Part model, mm, in its own coordinate system. A direction names the side the tool comes from. Coordinates: 2 decimals unless noted, no trailing zeros. Write each loop counter-clockwise with the first axis right and the second up, starting at its lowest first coordinate (ties: lowest second). Pieces come first, ordered by that corner, then holes. Notation, with made-up numbers: M 1,-4.5 L 15,-4.5 A25 ccw 15,31.5 Z; hole C 31.25,-5 d3. An arc over 180 degrees is marked long. Use a Markdown table: item, result. Add a question column.
Q1. Slice it at A-A on y = 0. Write the cut outline in (x, z), then the cut area to 3 significant figures.
Q2. Tool access for faces 1 (the flat face through (-29, -23.812, 5)), 2 (the flat face through (5, 38.1, 23)), 3 (the flat face through (18.149, 11.414, 5.478)), 4 (the flat face through (29, -23.812, 5)): list every direction of +Z, -Z, +X, -X, +Y, -Y with a clear straight run to the whole face (end or side of a thin tool).
Q3. Slice it at C-C on x = 8. Write the cut outline in (y, z), then the cut area to 3 significant figures.
Q4. Mould opens along X. For faces 5 (the cylindrical face through (-0.419, 44.361, 52.383)), 6 (the flat face through (34.925, -29, 5)), 7 (the flat face through (-2.63, 44.45, 38.43)) say: released by +X, released by -X, zero draft, split by the parting line, or undercut.
Q5. Pin check, flat tips, straight feed: pin 1 Ø12.5 at (y, z) = (38, 24.5) entering from +X; pin 2 Ø1 at (x, y) = (22, -2) entering from -Z; pin 3 Ø6 at (x, y) = (-13.5, 29) entering from +Z; pin 4 Ø24.5 at (x, z) = (5.5, 35.5) entering from -Y. Stop position of each tip, or through.
Q6. Wall check: L1, parallel to Z at x = 0, y = 48; L2, parallel to Z at x = 0, y = 40 (3 decimals); L3, parallel to Y at x = 0, z = 4. Give the ranges that are in metal, low to high. Write a range as from..to.
Q7. Slice it at B-B on x = 0. Count the separate pieces of the cut face and the enclosed holes in it, then the cut area to 3 significant figures.
from build123d import *

# Parameters (mm, degrees)
PAD_DEPTH       = 11.1125
PAD001_DEPTH    = 12.7
SKETCH002_R     = 11.1125
POCKET_DEPTH    = 6.35
SKETCH003_R     = 5.55625
POCKET001_DEPTH = 6.351


with BuildPart() as part:
    # Sketch → Pad (new body)
    with BuildSketch(Plane.XY):
        with BuildLine():
            ThreePointArc((4.957324, 11.692516), (-8.980256, -8.980256), (11.692516, 4.957324))
            Line((24.428163, 17.692971), (11.692516, 4.957324))
            ThreePointArc((23.688223, -18.672024), (30.156258, -0.613607), (24.428163, 17.692971))
            ThreePointArc((23.688223, -18.672024), (23.325058, -22.023177), (26.181706, -23.8125))
            Line((31.75, -23.8125), (26.181706, -23.8125))
            ThreePointArc((34.925, -26.9875), (33.995064, -24.742436), (31.75, -23.8125))
            Line((34.925, -31.75), (34.925, -26.9875))
            Line((-34.925, -31.75), (34.925, -31.75))
            Line((-34.925, -31.75), (-34.925, -26.9875))
            ThreePointArc((-31.75, -23.8125), (-33.995064, -24.742436), (-34.925, -26.9875))
            Line((-31.75, -23.8125), (-26.181706, -23.8125))
            ThreePointArc((-26.181706, -23.8125), (-23.325058, -22.023177), (-23.688223, -18.672024))
            ThreePointArc((-19.05, 23.385335), (-29.980732, 3.306373), (-23.688223, -18.672024))
            Line((-19.05, 23.385335), (-19.05, 38.1))
            Line((-19.05, 38.1), (19.05, 38.1))
            Line((19.05, 38.1), (19.05, 25.785192))
            Line((19.05, 25.785192), (4.957324, 11.692516))
        make_face()
    extrude(amount=PAD_DEPTH)

    # Sketch001 → Pad001 (new body)
    with BuildSketch(Plane(origin=(0, 38.1, 0), x_dir=(-1, 0, 0), z_dir=(0, 1, 0))):
        with BuildLine():
            Line((-19.05, 0), (19.05, 0))
            Line((19.05, 0), (19.05, 11.1125))
            Line((19.049953, 33.337541), (19.05, 11.1125))
            ThreePointArc((19.049953, 33.337541), (-2.3e-05, 52.387477), (-19.05, 33.337541))
            Line((-19.05, 33.337541), (-19.05, 11.1125))
            Line((-19.05, 0), (-19.05, 11.1125))
        make_face()
    extrude(amount=PAD001_DEPTH)

    # Sketch002 → Pocket (cut)
    with BuildSketch(Plane.XZ.offset(-38.1)):
        with Locations((0, 33.3375)):
            Circle(SKETCH002_R)
    extrude(amount=-POCKET_DEPTH, mode=Mode.SUBTRACT)

    # Sketch003 → Pocket001 (cut, through all)
    with BuildSketch(Plane.XZ.offset(-44.45)):
        with Locations((0, 33.3375)):
            Circle(SKETCH003_R)
    extrude(amount=-POCKET001_DEPTH, mode=Mode.SUBTRACT)


solid = part.part
Recorded:
| question | item | result |
|---|---|---|
| 1 | outline | M -30.16,0 L -12.7,0 L -12.7,11.11 L -30.16,11.11 Z; M 12.7,0 L 30.16,0 L 30.16,11.11 L 12.7,11.11 Z |
| 1 | area | 388 mm² |
| 2 | face 1 | +Z, -Z, -X |
| 2 | face 2 | +Z, +X, -X, -Y |
| 2 | face 3 | +Z, -Z |
| 2 | face 4 | +Z, -Z, +X |
| 3 | outline | M -31.75,0 L -9.86,0 L -9.86,11.11 L -31.75,11.11 Z; M 14.74,0 L 50.8,0 L 50.8,50.63 L 38.1,50.63 L 38.1,41.05 L 44.45,41.05 L 44.45,25.62 L 38.1,25.62 L 38.1,11.11 L 14.74,11.11 Z |
| 3 | area | 1,050 mm² |
| 4 | face 5 | split by the parting line |
| 4 | face 6 | released by +X |
| 4 | face 7 | undercut |
| 5 | pin 1 | x = 19.05 |
| 5 | pin 2 | z = 0 |
| 5 | pin 3 | z = 11.11 |
| 5 | pin 4 | y = 38.1 |
| 6 | L1 | 0..27.78, 38.89..52.39 |
| 6 | L2 | 0..22.225, 44.45..52.387 |
| 6 | L3 | -31.75..-12.7, 12.7..50.8 |
| 7 | separate pieces | 3 |
| 7 | enclosed holes | 0 |
| 7 | area | 948 mm² |
